Geometry: final body of the model. Coordinates: model frame, mm. Face numbers are marked on the shaded views. A direction names the side the tool comes from. Round coordinates to 2 decimals unless told otherwise and drop trailing zeros. Loops run counter-clockwise (first coordinate to the right, second up) from the corner with the lowest first, then second, coordinate; pieces in that order, holes last. Notation, with made-up numbers: (72.25, 20) - (86.25, 20) arc R31 cw to (86.25, 47) - close; hole circle Ø10 at (-25, 21.5). An arc over 180 degrees is marked (long way). Answer as a JSON object with one key per item and string values. Group by question number.
Item 1: First-contact query: pin 1 (8 mm diameter, centred on y = 279, z = -5.5, fed in from -X); pin 2 (2 mm diameter, centred on x = -2, y = 409.5, fed in from -Z); pin 3 (8 mm diameter, centred on x = 28, y = 251, fed in from +Z). Flat tips, straight axial feed; report the tip coordinate or a pass-through.
Item 2: Line query: line 1 (X direction, y = 161, z = 13); line 2 (X direction, y = 101.5, z = 42.5); line 3 (Y direction, x = 41, z = 6). Output: solid intervals per line, ascending.
Item 3: Section B-B (y = 379.5). Return the cut outline in (x, z), plus the area to 3 significant figures.
Item 4: Section A-A (y = 285). Return the cut outline in (x, z), plus the area to 3 significant figures.
Item 5: Reachability of the marked faces 1 and 2 from +Z, -Z, +X, -X, +Y, -Y: full face, straight path, thin tool, end or side. Return the list, or none.
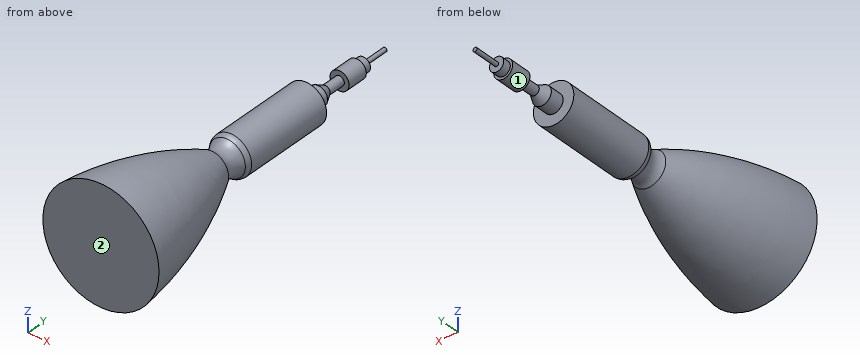
```python
from build123d import *

# Parameters (mm, degrees)
FILLET1_R = 10


with BuildPart() as part:
    # Sketch1 → Revolve1 (revolve)
    with BuildSketch(Plane.XY):
        with BuildLine():
            Line((0, 0), (76, 0))
            ThreePointArc((76, 0), (57.779229612, 91.871941274), (22.501351501, 178.635536076))
            ThreePointArc((22.501351501, 178.635536076), (18.690152094, 193.361033944), (26.407726548, 206.468458288))
            Line((26.407726548, 206.468458288), (26.407726548, 332))
            Line((26.407726548, 332), (0, 332))
            Line((0, 332), (0, 0))
        make_face()
    revolve(axis=Axis((0, 0, 0), (0, 1, 0)))

    # Fillet1
    fillet1_edges = [part.edges().sort_by_distance(p)[0] for p in [
        (-26.407726548, 206.468458288, 0),
    ]]
    fillet(fillet1_edges, radius=FILLET1_R)

    # Sketch2 → Revolve2 (revolve)
    with BuildSketch(Plane.XY):
        Polygon((0, 332), (0, 459), (2.664793977, 459), (2.664793977, 424.102348648), (9.322424203, 424.102348648), (9.322424203, 413.501049111), (12.429898937, 413.501049111), (12.429898937, 385.623557734), (6.214949468, 385.623557734), (6.214949468, 362.850395765), (12.429898937, 351.071174056), (12.429898937, 332), align=None)
    revolve(axis=Axis((0, 332, 0), (0, 1, 0)))


solid = part.part
```
Values:
{
 "1": {"pin 1": "stops at x = -26.37", "pin 2": "stops at z = -12.39", "pin 3": "stops at z = 11.02"},
 "2": {"line 1": "x = -28.44 to 28.44", "line 2": "x = -34.58 to 34.58", "line 3": "y = 0 to 137.98"},
 "3": {"outline": "circle Ø12.43 at (0, 0)", "area": "121 mm^2"},
 "4": {"outline": "circle Ø52.82 at (0, 0)", "area": "2,190 mm^2"},
 "5": {"face 1": "+Y", "face 2": "+Z, -Z, +X, -X, -Y"}
}
